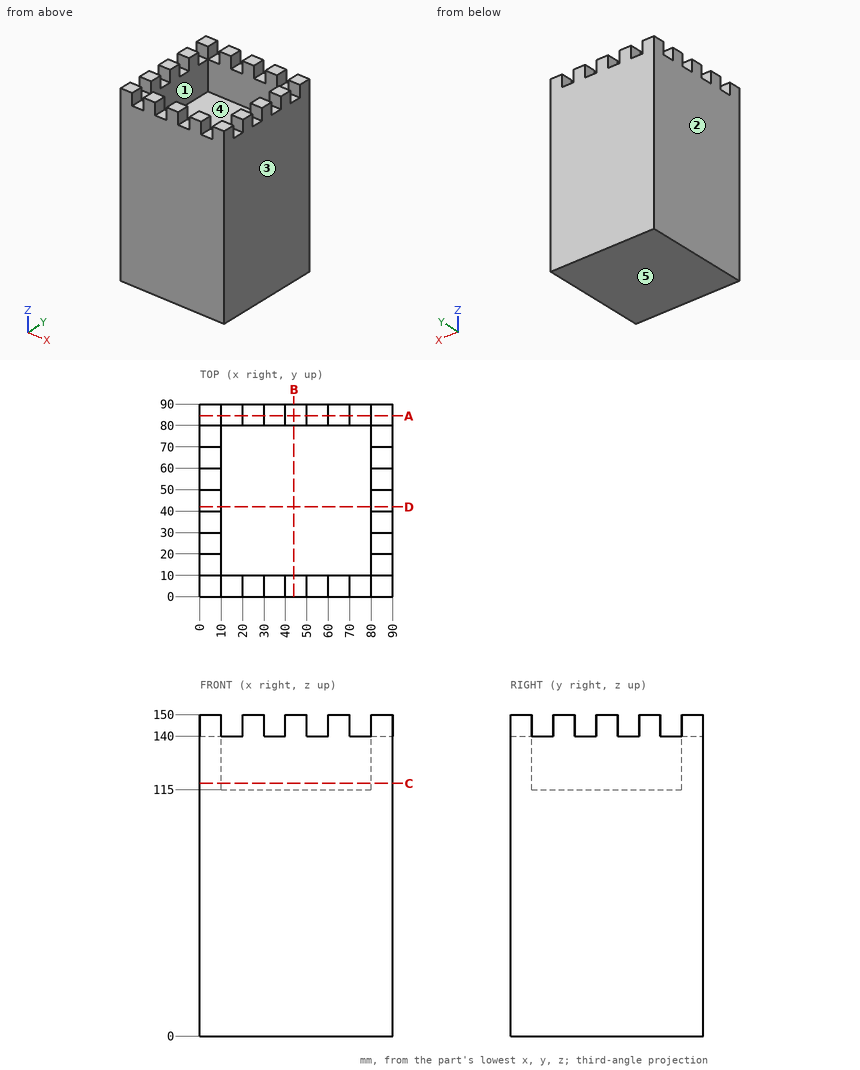
Geometry check sheet. Reference: drawing and pictorial views, mm from the part's lowest x, y, z. A direction names the side the tool comes from. Round coordinates to 2 decimals unless told otherwise and drop trailing zeros. Write each loop counter-clockwise with the first axis right and the second up, starting at its lowest first coordinate (ties: lowest second). Pieces come first, ordered by that corner, then holes.
1. Scan lines: L1, parallel to Y at x = 31, z = 124.5; L2, parallel to Z at x = 72.5, y = 69.5. Record each from-to range of solid material in increasing order.
2. Section check A-A on y = 84.5. Enter the section's corners in (x, z), plus the area to 3 significant figures.
3. Section check B-B on x = 44. Enter the section's corners in (y, z), plus the area to 4 significant figures.
4. Gauge pin test, flat ends, axial feed: P1, Ø5, axis at x = 53, y = 3, coming from the +Z side; P2, Ø4, axis at x = 50, y = 61, coming from the +Z side. Record the tip position at first contact, or that the pin passes through.
5. Draft check along X on the marked faces 3, 4 and 5. Enter one of: +X half, -X half, draft (parallel to the pull), parting line (faces both ways), or undercut.
6. Access from +Z, -Z, +X, -X, +Y, -Y to the whole of each face (thin tool, end or side, straight path). Record for the marked faces 1 and 2.
7. Section check C-C on z = 118. Enter the section's corners in (x, y).
Answer:
1. L1: y = 0 to 10, 80 to 90
1. L2: z = 0 to 115
2. outline: (0, 0) - (90, 0) - (90, 150) - (80, 150) - (80, 140) - (70, 140) - (70, 150) - (60, 150) - (60, 140) - (50, 140) - (50, 150) - (40, 150) - (40, 140) - (30, 140) - (30, 150) - (20, 150) - (20, 140) - (10, 140) - (10, 150) - (0, 150) - close
2. area: 13,100 mm2
3. outline: (0, 0) - (90, 0) - (90, 150) - (80, 150) - (80, 115) - (10, 115) - (10, 150) - (0, 150) - close
3. area: 11,050 mm2
4. P1: stops at z = 140
4. P2: stops at z = 115
5. face 3: +X half
5. face 4: undercut
5. face 5: draft
6. face 1: +Z
6. face 2: +Z, -Z, -X, +Y, -Y
7. outline: (0, 0) - (90, 0) - (90, 90) - (0, 90) - close; hole (10, 10) - (80, 10) - (80, 80) - (10, 80) - close
